from build123d import *

# Parameters (mm, degrees)
F1_DEPTH = 5
F3_R     = 2


# Not quite as in the source:
# - a feature of the source that left no trace in its solid (it failed there, or was rolled back) is left out
# - a feature names something its author has since deleted; it is built from what else it names


with BuildPart() as f1:
    # F0 (on Top) → F1 (new body)
    with BuildSketch(Plane.XY):
        with BuildLine():
            ThreePointArc((1, 4.2856675661), (0.9540832917, 3.9861261291), (0.820549855, 3.7140926057))
            ThreePointArc((0.820549855, 3.7140926057), (0.7011095464, 3.5726139889), (0.5576336696, 3.4555804077))
            Line((0.5576336696, 3.4555804077), (-3.5314378692, -0.5649969839))
            ThreePointArc((-3.5314378692, -0.5649969839), (-3.0925503087, -0.8559404108), (-2.6298440658, -1.1072834062))
            ThreePointArc((-2.6298440658, -1.1072834062), (0, -0.714485053), (2.6298440658, -1.1072834062))
            ThreePointArc((2.6298440658, -1.1072834062), (3.4591021242, -0.6168432696), (4.1991729558, 0))
            ThreePointArc((4.1991729558, 0), (5.531502406, 1.961343765), (6, 4.2856675661))
            ThreePointArc((6, 4.2856675661), (2.4042381835, 9.7829067602), (-4.073212919, 8.6912250242))
            Line((-4.073212919, 8.6912250242), (-4.3361291045, 8.4327128262))
            ThreePointArc((-4.3361291045, 8.4327128262), (-5.9823120662, 4.7460395278), (-4.9195913989, 0.8509011303))
            Line((-4.9195913989, 0.8509011303), (-0.7011096797, 4.9987210123))
            ThreePointArc((-0.7011096797, 4.9987210123), (0.3865813759, 5.2079228669), (1, 4.2856675661))
        make_face()
        with BuildLine():
            ThreePointArc((-2.6298440658, -1.1072834062), (-3.0925503087, -0.8559404108), (-3.5314378692, -0.5649969839))
            Line((-3.5314378692, -0.5649969839), (-6.3099859173, -3.297002858))
            ThreePointArc((-6.3099859173, -3.297002858), (-4.6020493099, -1.9800722021), (-2.6298440658, -1.1072834062))
        make_face()
        with BuildLine():
            Line((-7.7001872259, -1.8831182213), (-4.9195913989, 0.8509011303))
            ThreePointArc((-4.9195913989, 0.8509011303), (-5.9823120662, 4.7460395278), (-4.3361291045, 8.4327128262))
            Line((-4.3361291045, 8.4327128262), (-11.2037486913, 1.6801295606))
            Line((-11.2037486913, 1.6801295606), (-7.7001872259, -1.8831182213))
        make_face()
        with BuildLine():
            ThreePointArc((2.6298440658, -1.1072834062), (0, -0.714485053), (-2.6298440658, -1.1072834062))
            ThreePointArc((-2.6298440658, -1.1072834062), (0, -1.7143324339), (2.6298440658, -1.1072834062))
        make_face()
        with BuildLine():
            ThreePointArc((2.6298440658, -1.1072834062), (0, -1.7143324339), (-2.6298440658, -1.1072834062))
            ThreePointArc((-2.6298440658, -1.1072834062), (-4.6020493099, -1.9800722021), (-6.3099859173, -3.297002858))
            ThreePointArc((-6.3099859173, -3.297002858), (-6.4229942249, -16.018860136), (6.2987594337, -16.1429864022))
            Line((6.2987594337, -16.1429864022), (2.7994486372, -12.5715967638))
            ThreePointArc((2.7994486372, -12.5715967638), (-2.8571117107, -12.5139336903), (-2.7994486372, -6.8573733423))
            Line((-2.7994486372, -6.8573733423), (2.9592441197, -1.2149042257))
            ThreePointArc((2.9592441197, -1.2149042257), (2.7950621185, -1.1595082703), (2.6298440658, -1.1072834062))
        make_face()
        with BuildLine():
            ThreePointArc((4.1991729558, 0), (3.4591021242, -0.6168432696), (2.6298440658, -1.1072834062))
            ThreePointArc((2.6298440658, -1.1072834062), (2.7950621185, -1.1595082703), (2.9592441197, -1.2149042257))
            Line((2.9592441197, -1.2149042257), (4.1991729558, 0))
        make_face()
    extrude(amount=F1_DEPTH)

    # F3
    f3_edges = [f1.edges().sort_by_distance(p)[0] for p in [
        (-11.203749, 1.68013, 2.5),
        (-7.700187, -1.883118, 2.5),
        (6.298759, -16.142986, 2.5),
        (2.799449, -12.571597, 2.5),
    ]]
    fillet(f3_edges, radius=F3_R)


solid = f1.part
Geometry check sheet. Reference: the model listing, model coordinates, mm. A direction names the side the tool comes from. Give positions to 0.01 mm unless a question says otherwise; leave off trailing zeros. Loops run counter-clockwise (first coordinate to the right, second up) from the corner with the lowest first, then second, coordinate; pieces in that order, holes last. Notation, with made-up numbers: (88, -19) -> (147, -19) arc R28 ccw to (147, 16) -> close; hole circle Ø3 at (62, 46.5). An arc over 180 degrees is marked (long way). Answer in a Markdown table with one row per item. Add a question column.
1) Cross-section at D-D on z = 0.7. Record the boundary of the cut face in (x, y) (3 decimals).
2) Set-up check for faces 1 (the face through (5.24, -16.24, 2.54)), 2 (the face through (-7.715, -1.054, 2.535)): record each of +Z, -Z, +X, -X, +Y, -Y from which the full face is reachable in a straight line by a thin tool's end or side.
3) Cross-section at B-B on x = -1. Record the boundary of the cut face in (y, z), and give its area (3 significant figures).
4) Cross-section at A-A on y = 1.5. Record the boundary of the cut face in (x, z), and give its area (3 significant figures).
5) Material ranges on probe 1 along Y at (x, z) = (0.25, 0.25); probe 2 along Y at (x, z) = (-3, 1.7); probe 3 along Y at (x, z) = (-8, 1.75), recorded low to high. Write a range as from..to.
6) Cross-section at C-C on x = -8. Record the boundary of the cut face in (y, z).
7) Gauge pin test, flat ends, axial feed: P1, Ø2, axis at x = -3.5, z = 4.5, coming from the +Y side; P2, Ø3, axis at y = -4.5, z = 2, coming from the -X side. Record the tip position at first contact, or that the pin passes through.
8) Draft check along Y on faces 3 (the face through (-10.375, 1.695, 2.535)), 4 (the face through (-7.37, -14.88, 2.46)), 5 (the face through (2.91, -13.19, 2.54)), 6 (the face through (-2, -4, 0)). Enter one of: pulls with the +Y half, pulls with the -Y half, needs draft (parallel to the pull), parting line crosses it, or undercut.
Outcome:
| question | item | result |
|---|---|---|
| 1 | outline | (-9.802, 0.254) -> (-9.102, -0.457) arc R2 ccw to (-6.274, -0.481) -> (-0.701, 4.999) arc R1 cw (long way) to (0.558, 3.456) -> (-6.31, -3.297) arc R9 ccw to (4.199, -17.675) arc R2 ccw to (4.695, -14.506) -> (3.959, -13.755) arc R2 ccw to (1.687, -13.341) arc R4 cw to (-2.799, -6.857) -> (4.199, 0) arc R6 ccw to (-4.073, 8.691) -> (-9.778, 3.082) arc R2 ccw to start |
| 2 | face 1 | +Z, -Z, +X |
| 2 | face 2 | +Z, -Z |
| 3 | outline | (-18.66, 0) -> (-13.59, 0) -> (-13.59, 5) -> (-18.66, 5) -> close; (-5.09, 0) -> (1.92, 0) -> (1.92, 5) -> (-5.09, 5) -> close; (4.7, 0) -> (10.2, 0) -> (10.2, 5) -> (4.7, 5) -> close |
| 3 | area | 87.9 mm^2 |
| 4 | outline | (-10.37, 0) -> (-4.26, 0) -> (-4.26, 5) -> (-10.37, 5) -> close; (-1.43, 0) -> (5.31, 0) -> (5.31, 5) -> (-1.43, 5) -> close |
| 4 | area | 64.3 mm^2 |
| 5 | probe 1 | y = -18.71..-13.71, -3.87..3.15, 5.25..10.28 |
| 5 | probe 2 | y = -18.2..-12.36, -7.07..-0.04, 2.74..9.48 |
| 5 | probe 3 | y = -13.84..-5.59, -1.03..4.83 |
| 6 | outline | (-13.84, 0) -> (-5.59, 0) -> (-5.59, 5) -> (-13.84, 5) -> close; (-1.03, 0) -> (4.83, 0) -> (4.83, 5) -> (-1.03, 5) -> close |
| 7 | P1 | stops at y = 9.74 |
| 7 | P2 | stops at x = -8.2 |
| 8 | face 3 | parting line crosses it |
| 8 | face 4 | undercut |
| 8 | face 5 | undercut |
| 8 | face 6 | needs draft |
